The figure shows three views and two pictorial views of one solid part (mm, origin at its lowest corner). Answer the questions. A direction names the side the tool comes from. Give positions to 0.01 mm unless a question says otherwise; leave off trailing zeros. Write each loop counter-clockwise with the first axis right and the second up, starting at its lowest first coordinate (ties: lowest second). Pieces come first, ordered by that corner, then holes. Notation, with made-up numbers: (28.25, 61) - (58.25, 61) arc R25 ccw to (58.25, 100) - close; hole circle Ø2 at (72.5, -25.75). An arc over 180 degrees is marked (long way). One line per question, with ' | ' between items. Start each with the question number.
1. The mould has two halves that part along X. Classify the marked faces 3, 4 and 5: +X half, -X half, draft (parallel to the pull), parting line (faces both ways), or undercut.
2. A cutting plane is placed at A-A (z = 6.5). Determine the outline of the cut face in (x, y), then the cut area to 3 significant figures.
3. A cutting plane is placed at B-B (y = 12.25). Determine the outline of the cut face in (x, z), then the cut area to 3 significant figures.
4. Given P1, Ø1, axis at x = 3.5, y = 3.5, coming from the -Z side; P2, Ø1, axis at x = 3.5, z = 10.5, coming from the +Y side; P3, Ø1, axis at x = 10, y = 3.5, coming from the +Z side, each flat-ended and moving along its own axis, determine where each tip first touches the part or whether it passes through.
5. Find the intervals of material crossed by L1, parallel to Y at x = 3.5, z = 6.5; L2, parallel to Y at x = 12.75, z = 6.5; L3, parallel to X at y = 1.5, z = 9, in increasing order. Write a range as from..to.
6. A cutting plane is placed at C-C (x = 12.25). Determine the outline of the cut face in (y, z).
7. For the marked faces 1 and 2, determine the directions among +Z, -Z, +X, -X, +Y, -Y from which every point of the face is accessible in a straight line to the end or side of a thin tool.
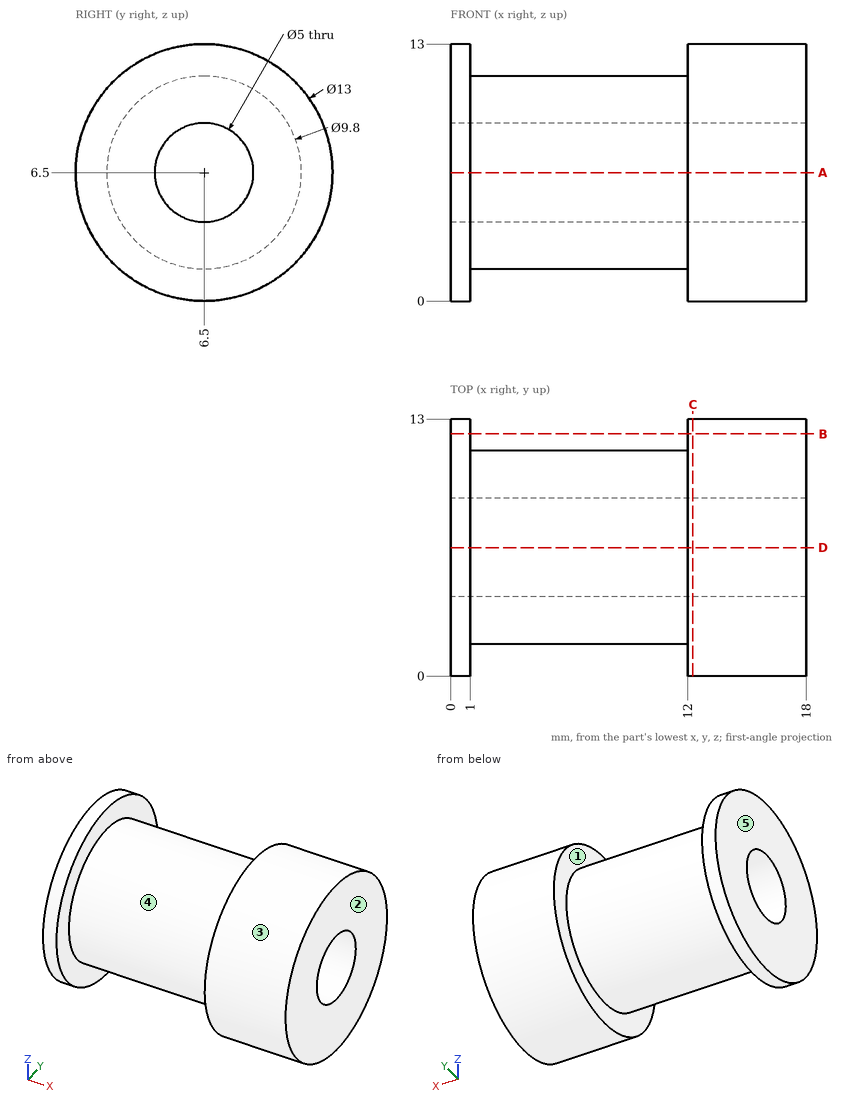
Determined:
1) face 3: draft | face 4: undercut | face 5: -X half
2) outline: (0, 0) - (1, 0) - (1, 1.6) - (12, 1.6) - (12, 0) - (18, 0) - (18, 4) - (0, 4) - close; (0, 9) - (18, 9) - (18, 13) - (12, 13) - (12, 11.4) - (1, 11.4) - (1, 13) - (0, 13) - close | area: 109 mm2
3) outline: (0, 3.47) - (1, 3.47) - (1, 9.53) - (0, 9.53) - close; (12, 3.47) - (18, 3.47) - (18, 9.53) - (12, 9.53) - close | area: 42.4 mm2
4) P1: z = 2.29 | P2: y = 9.93 | P3: z = 10.71
5) L1: 1.6..4, 9..11.4 | L2: 0..4, 9..13 | L3: 0..1, 12..18
6) outline: circle Ø13 at (6.5, 6.5); hole circle Ø5 at (6.5, 6.5)
7) face 1: none | face 2: +Z, -Z, +X, +Y, -Y
